Geometry check sheet. Reference: drawing and pictorial views, mm from the part's lowest x, y, z. Coordinates: 2 decimals unless noted, no trailing zeros. Loops run counter-clockwise (first coordinate to the right, second up) from the corner with the lowest first, then second, coordinate; pieces in that order, holes last. Notation, with made-up numbers: M -10,46.5 L 1,46.5 A19 cw 1,78.5 Z; hole C 67,31 d3. An arc over 180 degrees is marked long. Write item = value, one per line. Start each with the question number.
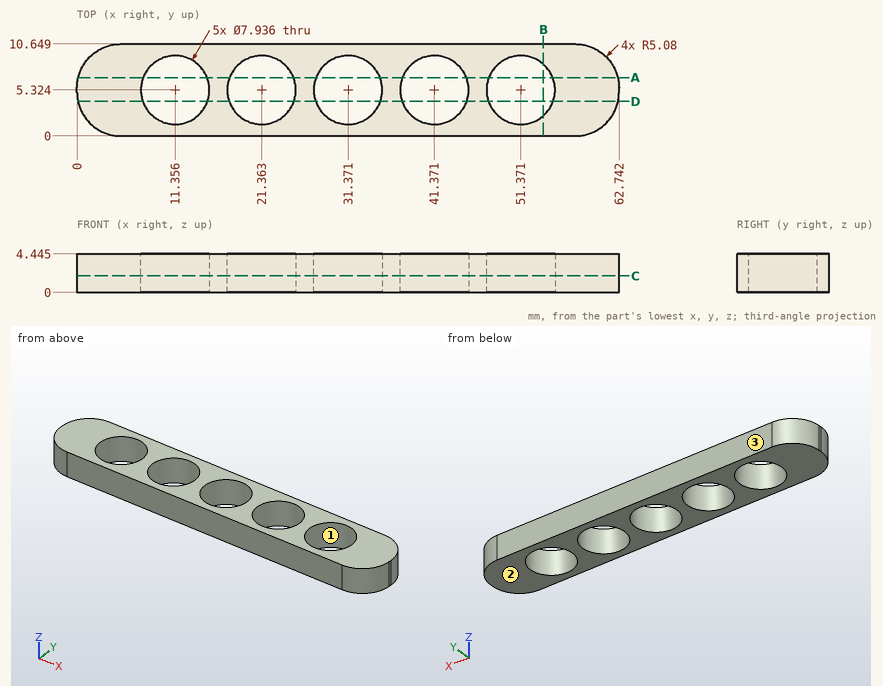
Q1. Gauge pin test, flat ends, axial feed: pin 1 (1.5 mm diameter, centred on y = 3, z = 1.5, fed in from +X) (1 decimal); pin 2 (3 mm diameter, centred on x = 13, y = 6, fed in from -Z) (3 decimals); pin 3 (1.5 mm diameter, centred on y = 1.5, z = 1, fed in from +X). Record the tip position at first contact, or that the pin passes through.
Q2. Scan lines: L1, parallel to Y at x = 21.5, z = 2.45; L2, parallel to X at y = 3, z = 1.7 (1 decimal); L3, parallel to X at y = 6.25, z = 1.5 (1 decimal). Record each from-to range of solid material in increasing order. Write a range as [from, to].
Q3. Sectioned sample at B-B on x = 54. Record the cut outline in (y, z) (1 decimal), plus the area to 3 significant figures.
Q4. Sectioned sample at C-C on z = 1.9. Record the cut outline in (x, y) (1 decimal).
Q5. Mould release check, pull along Y, two halves, no side actions. Record for the marked faces 1, 2 and 3: +Y half, -Y half, draft (parallel to the pull), parting line (faces both ways), or undercut.
Q6. Sectioned sample at D-D on y = 4. Record the cut outline in (x, z) (1 decimal), plus the area to 3 significant figures.
Q7. Sectioned sample at A-A on y = 6.75. Record the cut outline in (x, z) (1 decimal), plus the area to 3 significant figures.
Solutions:
q1.pin_1 = 62.6
q1.pin_2 = through
q1.pin_3 = 61.88
q2.L1 = [0, 1.36], [9.29, 10.65]
q2.L2 = [0.4, 8.1], [14.6, 18.1], [24.6, 28.2], [34.6, 38.2], [44.6, 48.2], [54.6, 62.3]
q2.L3 = [0, 7.5], [15.2, 17.5], [25.2, 27.5], [35.2, 37.5], [45.2, 47.5], [55.2, 62.7]
q3.outline = M 0,0 L 2.4,0 L 2.4,4.4 L 0,4.4 Z; M 8.3,0 L 10.6,0 L 10.6,4.4 L 8.3,4.4 Z
q3.area = 20.9 mm²
q4.outline = M 0,5.1 A5.1 ccw 5.1,0 L 57.7,0 A5.1 ccw 62.7,5.1 L 62.7,5.6 A5.1 ccw 57.7,10.6 L 5.1,10.6 A5.1 ccw 0,5.6 Z; hole C 11.4,5.3 d7.9; hole C 21.4,5.3 d7.9; hole C 31.4,5.3 d7.9; hole C 41.4,5.3 d7.9; hole C 51.4,5.3 d7.9
q5.face_1 = undercut
q5.face_2 = draft
q5.face_3 = +Y half
q6.outline = M 0.1,0 L 7.6,0 L 7.6,4.4 L 0.1,4.4 Z; M 15.1,0 L 17.6,0 L 17.6,4.4 L 15.1,4.4 Z; M 25.1,0 L 27.6,0 L 27.6,4.4 L 25.1,4.4 Z; M 35.1,0 L 37.6,0 L 37.6,4.4 L 35.1,4.4 Z; M 45.1,0 L 47.6,0 L 47.6,4.4 L 45.1,4.4 Z; M 55.1,0 L 62.6,0 L 62.6,4.4 L 55.1,4.4 Z
q6.area = 112 mm²
q7.outline = M 0.1,0 L 7.7,0 L 7.7,4.4 L 0.1,4.4 Z; M 15.1,0 L 17.7,0 L 17.7,4.4 L 15.1,4.4 Z; M 25.1,0 L 27.7,0 L 27.7,4.4 L 25.1,4.4 Z; M 35.1,0 L 37.7,0 L 37.7,4.4 L 35.1,4.4 Z; M 45.1,0 L 47.7,0 L 47.7,4.4 L 45.1,4.4 Z; M 55.1,0 L 62.6,0 L 62.6,4.4 L 55.1,4.4 Z
q7.area = 113 mm²
